Could you check a few things on this model? Use its own coordinates, in mm. A direction names the side the tool comes from. Coordinates: 2 decimals unless noted, no trailing zeros. Write each loop counter-clockwise with the first axis right and the second up, starting at its lowest first coordinate (ties: lowest second). Pieces come first, ordered by that corner, then holes. Notation, with made-up numbers: (-20, 54) - (-7, 54) arc R16 cw to (-7, 61) - close; hole circle Ø11 at (59, 52). An arc over 180 degrees is marked (long way). Write item = value, one per line. Start each with the question number.
```python
from build123d import *

# Parameters (mm, degrees)
SKETCH_W        = 52
SKETCH_H        = 52
PAD_DEPTH       = 5
SKETCH005_R     = 3.5
PAD001_DEPTH    = 1.5
SKETCH001_R     = 12.5
SKETCH001_R_2   = 1.8
POCKET_DEPTH    = 6.501
SKETCH006_R     = 3.7
POCKET001_DEPTH = 2.5


with BuildPart() as part:
    # Sketch → Pad (new body)
    with BuildSketch(Plane.XY):
        Rectangle(SKETCH_W, SKETCH_H)
    extrude(amount=PAD_DEPTH)

    # Sketch005 → Pad001 (new body)
    with BuildSketch(Plane.XY.offset(5)):
        with Locations((-18.5, -12.5)):
            Circle(SKETCH005_R)
        with Locations((18.5, -12.5)):
            Circle(SKETCH005_R)
    extrude(amount=PAD001_DEPTH)

    # Sketch001 → Pocket (cut, through all)
    with BuildSketch(Plane(origin=(0, 0, 0), x_dir=(1, 0, 0), z_dir=(0, 0, -1))):
        Circle(SKETCH001_R)
        with Locations((0, 18.3)):
            Circle(SKETCH001_R_2)
        with Locations((0, -18.3)):
            Circle(SKETCH001_R_2)
        with Locations((-18.3, 0)):
            Circle(SKETCH001_R_2)
        with Locations((18.3, 0)):
            Circle(SKETCH001_R_2)
        with Locations((-18.5, 12.5)):
            Circle(SKETCH001_R_2)
        with Locations((18.5, 12.5)):
            Circle(SKETCH001_R_2)
        Polygon((-26, 4), (0, -22.037422), (26.037481, 3.962637), (26.037481, -34), (-26, -34), align=None)
    extrude(amount=-POCKET_DEPTH, mode=Mode.SUBTRACT)

    # Sketch006 → Pocket001 (cut)
    with BuildSketch(Plane(origin=(0, 0, 0), x_dir=(1, 0, 0), z_dir=(0, 0, -1))):
        with Locations((-18.3, 0)):
            Circle(SKETCH006_R)
        with Locations((0, 18.3)):
            Circle(SKETCH006_R)
        with Locations((18.3, 0)):
            Circle(SKETCH006_R)
        with Locations((0, -18.3)):
            Circle(SKETCH006_R)
    extrude(amount=-POCKET001_DEPTH, mode=Mode.SUBTRACT)


solid = part.part
```
1) Which directions (+Z, -Z, +X, -X, +Y, -Y) give clear straight access to the entire face, cutting with the end or side of a thin tool? Please do faces 5 (the cylindrical face through (-16.583, -0.541, 3.732)), 6 (the cylindrical face through (3.53, -19.41, 1.23)), 7 (the cylindrical face through (-16.885, -15.605, 5.74)).
2) Thinking about a two-plate mould opening in Y: for faces 1 (the cylindrical face through (20.017, -0.541, 3.732)), 2 (the flat face through (12.818, 9.238, 2.465)), 3 (the flat face through (26, -15, 2)), 4 (the cylindrical face through (18.266, -14.285, 3.204)), which applies, +Y half, -Y half, draft (parallel to the pull), parting line (faces both ways), or undercut?
3) Suppose I cut it at D-D on z = 3.5. Please give me the cut outline in (x, y), plus the area to 3 significant figures.
4) If I drill on probe 1 along X at (y, z) = (-18.3, 2.05); probe 2 along Y at (x, z) = (18.3, 3.7); probe 3 along X at (y, z) = (0, 4.05), over which ranges is the centre line in solid material (lowest first)? Write a range as [from, to].
5) Suppose I cut it at B-B on z = 0.75. Please give me the cut outline in (x, y).
6) For P1, Ø3.5, axis at x = -0.5, y = -19, coming from the -Z side; P2, Ø5, axis at x = 11.5, y = -15, coming from the +Z side; P3, Ø2, axis at y = -2, z = 2, coming from the +X side, each with a flat end and sliding along its axis, tell me the tip position at first contact or that it passes through.
7) Suppose I cut it at C-C on x = 7.5. Please give me the cut outline in (y, z), plus the area to 3 significant figures.
8) Suppose I cut it at A-A on y = -18.3. Please give me the cut outline in (x, z), plus the area to 4 significant figures.
Reply:
q1.face_5 = +Z, -Z
q1.face_6 = -Z
q1.face_7 = +Z
q2.face_1 = undercut
q2.face_2 = +Y half
q2.face_3 = draft
q2.face_4 = undercut
q3.outline = (-26, -26) - (26, -26) - (26, -3.93) - (0, 22.04) - (-26, -4) - close; hole circle Ø3.6 at (-18.5, -12.5); hole circle Ø3.6 at (-18.3, 0); hole circle Ø25 at (0, 0); hole circle Ø3.6 at (0, -18.3); hole circle Ø3.6 at (0, 18.3); hole circle Ø3.6 at (18.3, 0); hole circle Ø3.6 at (18.5, -12.5)
q3.area = 1,270 mm^2
q4.probe_1 = [-26, -3.7], [3.7, 26]
q4.probe_2 = [-26, -14.29], [-10.71, -1.8], [1.8, 3.76]
q4.probe_3 = [-22.01, -20.1], [-16.5, -12.5], [12.5, 16.5], [20.1, 22.07]
q5.outline = (-26, -26) - (26, -26) - (26, -3.93) - (22, 0.07) arc R3.7 cw (long way) to (18.36, 3.7) - (3.7, 18.34) arc R3.7 cw (long way) to (-3.7, 18.33) - (-18.31, 3.7) arc R3.7 cw (long way) to (-22, 0.01) - (-26, -4) - close; (-0.04, 22) arc R3.7 cw to (0.04, 22) - (0, 22.04) - close; hole circle Ø3.6 at (-18.5, -12.5); hole circle Ø25 at (0, 0); hole circle Ø7.4 at (0, -18.3); hole circle Ø3.6 at (18.5, -12.5)
q6.P1 = 2.5
q6.P2 = 5
q6.P3 = 25.07
q7.outline = (-26, 0) - (-10, 0) - (-10, 5) - (-26, 5) - close; (10, 0) - (14.55, 0) - (14.55, 5) - (10, 5) - close
q7.area = 103 mm^2
q8.outline = (-26, 0) - (-3.7, 0) - (-3.7, 2.5) - (-1.8, 2.5) - (-1.8, 5) - (-26, 5) - close; (1.8, 2.5) - (3.7, 2.5) - (3.7, 0) - (26, 0) - (26, 5) - (1.8, 5) - close
q8.area = 232.5 mm^2
